from build123d import *

# Parameters (mm, degrees)
CYLINDER022_R     = 15
CYLINDER022_DEPTH = 4


with BuildPart() as cono_brazo_central_base:
    # Cone → Cone (revolve)
    with BuildSketch(Plane(origin=(71.5, 2.5, 27), x_dir=(1, 0, 0), z_dir=(0, 1, 0))):
        Polygon((0, 0), (3, 0), (5.5, 21), (0, 21), align=None)
    revolve(axis=Axis((71.5, 2.5, 27), (0, 0, -1)))


with BuildPart() as union_base_brazo_central:
    # Cylinder022 → Cylinder022 (new body)
    with BuildSketch(Plane(origin=(71.5, 2.5, 5), x_dir=(1, 0, 0), z_dir=(0, 0, 1))):
        Circle(CYLINDER022_R)
    extrude(amount=CYLINDER022_DEPTH)

    # Fusion015: union Cono brazo central/base
    add(cono_brazo_central_base.part)


solid = union_base_brazo_central.part
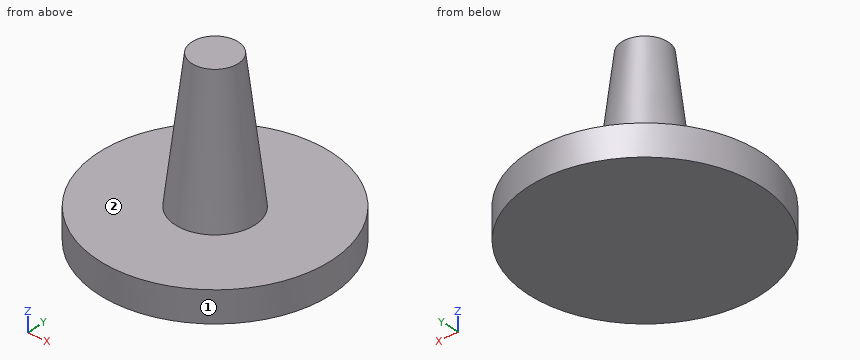
CAD build for the part. Positions are in the model's coordinates, mm. Face numbers are marked on the shaded views. A direction names the side the tool comes from. Coordinates: 2 decimals unless noted, no trailing zeros. Order: outer loops, then holes, each group sorted by start corner. A loop starts at its lowest first (then second) coordinate and runs counter-clockwise, first axis right, second up.
Item 1: Drill centre lines: L1, parallel to Z at x = 58.25, y = 2.5; L2, parallel to Y at x = 71.5, z = 7; L3, parallel to X at y = 5.5, z = 11.25. Where is each one in solid material? Low to high.
Check sheet entries:
L1: z = 5 to 9
L2: y = -12.5 to 17.5
L3: x = 67.66 to 75.34
Item 2: Band-saw the part on A-A on y = 2.5. List the corners of the cut face in (x, z), plus the area to 3 significant figures.
Check sheet entries:
outline: (56.5, 5) - (86.5, 5) - (86.5, 9) - (76.64, 9) - (74.5, 27) - (68.5, 27) - (66.36, 9) - (56.5, 9) - close
area: 267 mm2
Item 3: Band-saw the part on D-D on y = -6.5. List the corners of the cut face in (x, z), plus the area to 3 significant figures.
Check sheet entries:
outline: (59.5, 5) - (83.5, 5) - (83.5, 9) - (59.5, 9) - close
area: 96.0 mm2
Item 4: 3-axis set-ups, long thin cutter, end or side, ignore diameter. For the marked faces 1 and 2: which of +Z, -Z, +X, -X, +Y, -Y reach the whole face in a straight line?
Check sheet entries:
face 1: +Z, -Z
face 2: +Z
Item 5: Pin check, flat tips, straight feed: pin 1 Ø4 at (x, z) = (74, 23) entering from +Y; pin 2 Ø8 at (x, z) = (75, 15.5) entering from +Y; pin 3 Ø6 at (y, z) = (1, 18.5) entering from -X. Stop position of each tip, or through.
Check sheet entries:
pin 1: stops at y = 6.01
pin 2: stops at y = 7.16
pin 3: stops at x = 67.17
Item 6: Band-saw the part on B-B on x = 71.5. List the corners of the cut face in (y, z), plus the area to 3 significant figures.
Check sheet entries:
outline: (-12.5, 5) - (17.5, 5) - (17.5, 9) - (7.64, 9) - (5.5, 27) - (-0.5, 27) - (-2.64, 9) - (-12.5, 9) - close
area: 267 mm2
Item 7: Band-saw the part on C-C on z = 8.5. List the corners of the cut face in (x, y), plus the area to 3 significant figures.
Check sheet entries:
outline: circle Ø30 at (71.5, 2.5)
area: 707 mm2
